Here's how the part is built. I have some questions about the finished solid (model axes, mm). A direction names the side the tool comes from. Round coordinates to 2 decimals unless told otherwise and drop trailing zeros. Write each loop counter-clockwise with the first axis right and the second up, starting at its lowest first coordinate (ties: lowest second). Pieces come first, ordered by that corner, then holes. Notation, with made-up numbers: (34, 33.5) -> (41, 33.5) arc R10 ccw to (41, 40.5) -> close; hole circle Ø2 at (-33, 45). An arc over 180 degrees is marked (long way). Answer in a Markdown table with one row per item.
from build123d import *

# Parameters (mm, degrees)
SKETCH_1_R          = 50
EXTRUDE_1_DEPTH     = 5
SKETCH_5_R          = 2.75
CUT_EXTRUDE_4_DEPTH = 24
SKETCH_6_R          = 7.5
CUT_EXTRUDE_5_DEPTH = 24
SKETCH_7_R          = 2.4
CUT_EXTRUDE_6_DEPTH = 3


with BuildPart() as part:
    # 草图1 → 凸台-拉伸1 (new body)
    with BuildSketch(Plane(origin=(0, 0, 0), x_dir=(1, 0, 0), z_dir=(0, 1, 0))):
        with Locations(Location((0, 0, 0), (0, 0, 270))):
            Circle(SKETCH_1_R)
    extrude(amount=-EXTRUDE_1_DEPTH)

    # 草图5 → 切除-拉伸4 (cut)
    with BuildSketch(Plane(origin=(0, 0, 0), x_dir=(1, 0, 0), z_dir=(0, 1, 0))):
        with Locations(Location((28.284271247, 28.284271247, 0), (0, 0, 270))):
            Circle(SKETCH_5_R)
        with Locations(Location((28.284271247, -28.284271247, 0), (0, 0, 270))):
            Circle(SKETCH_5_R)
        with Locations(Location((-28.284271247, -28.284271247, 0), (0, 0, 270))):
            Circle(SKETCH_5_R)
        with Locations(Location((-28.284271247, 28.284271247, 0), (0, 0, 270))):
            Circle(SKETCH_5_R)
    extrude(amount=-CUT_EXTRUDE_4_DEPTH, mode=Mode.SUBTRACT)

    # 草图6 → 切除-拉伸5 (cut)
    with BuildSketch(Plane(origin=(0, 0, 0), x_dir=(1, 0, 0), z_dir=(0, 1, 0))):
        with Locations(Location((0, -28.284271247, 0), (0, 0, 270))):
            Circle(SKETCH_6_R)
    extrude(amount=-CUT_EXTRUDE_5_DEPTH, mode=Mode.SUBTRACT)

    # 草图7 → 切除-拉伸6 (cut)
    with BuildSketch(Plane(origin=(0, 0, 0), x_dir=(1, 0, 0), z_dir=(0, 1, 0))):
        with Locations(Location((40, 0, 0), (0, 0, 270))):
            Circle(SKETCH_7_R)
        with Locations(Location((0, 40, 0), (0, 0, 270))):
            Circle(SKETCH_7_R)
        with Locations(Location((-40, 0, 0), (0, 0, 270))):
            Circle(SKETCH_7_R)
    extrude(amount=-CUT_EXTRUDE_6_DEPTH, mode=Mode.SUBTRACT)


solid = part.part
1) I want a section at A-A, the plane x = 40. List the corners of the cut face in (y, z) for me, and give its area (3 significant figures).
Response:
| item | result |
|---|---|
| outline | (-5, -30) -> (0, -30) -> (0, -2.4) -> (-3, -2.4) -> (-3, 2.4) -> (0, 2.4) -> (0, 30) -> (-5, 30) -> close |
| area | 286 mm^2 |
2) For pin 1 (2.5 mm diameter, centred on x = 0.5, z = -40.5, fed in from +Y); pin 2 (4.5 mm diameter, centred on x = 28.28, z = 28.28, fed in from +Y); pin 3 (2 mm diameter, centred on y = -2, z = -5, fed in from -X); pin 4 (1 mm diameter, centred on x = 34, y = -2, fed in from -Z), each with a flat end and sliding along its axis, tell me the tip position at first contact or that it passes through.
Response:
| item | result |
|---|---|
| pin 1 | stops at y = -3 |
| pin 2 | passes through |
| pin 3 | stops at x = -49.84 |
| pin 4 | stops at z = -37.12 |
3) Which directions (+Z, -Z, +X, -X, +Y, -Y) give clear straight access to the entire face, cutting with the end or side of a thin tool? Please do faces 1 (the face through (-2.9, -2.5, 35.2)), 2 (the face through (0, -3, -40)).
Response:
| item | result |
|---|---|
| face 1 | +Y, -Y |
| face 2 | +Y |
4) I want a section at B-B, the plane z = -40. List the corners of the cut face in (x, y) for me, and give its area (3 significant figures).
Response:
| item | result |
|---|---|
| outline | (-30, -5) -> (30, -5) -> (30, 0) -> (2.4, 0) -> (2.4, -3) -> (-2.4, -3) -> (-2.4, 0) -> (-30, 0) -> close |
| area | 286 mm^2 |
5) We'd pull the mould along X, two halves only. Please class faces 3 (the face through (40, -3, 0)), 4 (the face through (15.02, -2.46, 47.69)), 5 (the face through (1, 0, -1)): +X half, -X half, draft (parallel to the pull), parting line (faces both ways), or undercut.
Response:
| item | result |
|---|---|
| face 3 | undercut |
| face 4 | parting line |
| face 5 | draft |
6) I want a section at C-C, the plane y = -1.8. Count the separate pieces of the cut face and the enclosed holes in it, and give its area (3 significant figures).
Response:
| item | result |
|---|---|
| separate pieces | 1 |
| enclosed holes | 8 |
| area | 7,530 mm^2 |
7) I want a section at D-D, the plane z = 0. List the corners of the cut face in (x, y) for me.
Response:
| item | result |
|---|---|
| outline | (-50, -5) -> (50, -5) -> (50, 0) -> (42.4, 0) -> (42.4, -3) -> (37.6, -3) -> (37.6, 0) -> (-37.6, 0) -> (-37.6, -3) -> (-42.4, -3) -> (-42.4, 0) -> (-50, 0) -> close |
8) I need wall thicknesses on line 1 (X direction, y = -1.05, z = 0); line 2 (Z direction, x = 28.5, y = -2.2); line 3 (X direction, y = -2.75, z = -29). Which ranges of each line are inside material? Lowest first, please. Write a range as [from, to].
Response:
| item | result |
|---|---|
| line 1 | x = [-50, -42.4], [-37.6, 37.6], [42.4, 50] |
| line 2 | z = [-41.08, -31.03], [-25.54, 25.54], [31.03, 41.08] |
| line 3 | x = [-40.73, -30.94], [-25.63, 25.63], [30.94, 40.73] |
